Here's the drawing with two shaded views (mm, measured from the low corner). I have some questions. A direction names the side the tool comes from. Coordinates: 2 decimals unless noted, no trailing zeros. Write each loop counter-clockwise with the first axis right and the second up, starting at its lowest first coordinate (ties: lowest second). Pieces come first, ordered by that corner, then holes. Notation, with made-up numbers: M 75.25,-31.75 L 133.25,-31.75 A27 ccw 133.25,4.25 Z; hole C 56,68.5 d3. An arc over 180 degrees is marked long. Answer as CSV lines item,"result". Start each with the question number.
Item 1: Suppose I cut it at A-A, the plane z = 12.5. Write out the boundary of the cut face in (x, y).
Item 2: Suppose I cut it at C-C, the plane y = 9. Write out the boundary of the cut face in (x, z).
Item 3: If I drill on line 1 along X through (y, z) = (35, 15.25); line 2 along Y through (x, z) = (22.5, 8.5), over which ranges is the centre line in solid material (lowest first)? Write a range as [from, to].
Item 4: Suppose I cut it at D-D, the plane x = 22.5. Write out the boundary of the cut face in (y, z).
Item 5: On a 3-axis mill with a long thin cutter (end or side, diameter ignored), from which of +Z, -Z, +X, -X, +Y, -Y can I reach the whole of each face in a straight line? I mean the marked faces 1 and 2. Say none if no direction works.
Item 6: I'm going to push flat-ended pins straight in: P1, Ø17.5, axis at x = 19, y = 19, coming from the +Z side; P2, Ø1, axis at x = 38.5, y = 10, coming from the +Z side. Where does each tip first touch, or does it pass through?
Item 7: Suppose I cut it at B-B, the plane z = 17.5. Write out the boundary of the cut face in (x, y).
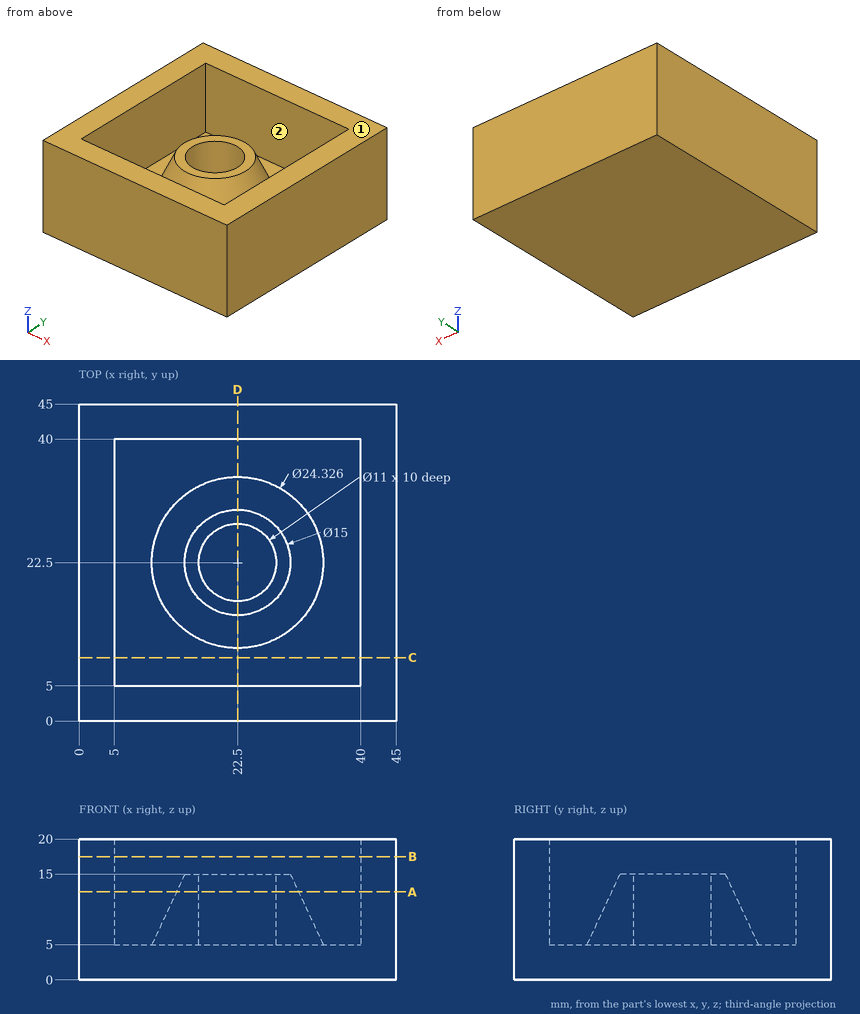
Ans:
1,outline,"M 0,0 L 45,0 L 45,45 L 0,45 Z; C 22.5,22.5 d17.33; hole M 5,5 L 40,5 L 40,40 L 5,40 Z; hole C 22.5,22.5 d11"
2,outline,"M 0,0 L 45,0 L 45,20 L 40,20 L 40,5 L 5,5 L 5,20 L 0,20 Z"
3,line 1,"x = [0, 5], [40, 45]"
3,line 2,"y = [0, 5], [11.97, 17], [28, 33.03], [40, 45]"
4,outline,"M 0,0 L 45,0 L 45,20 L 40,20 L 40,5 L 34.66,5 L 30,15 L 28,15 L 28,5 L 17,5 L 17,15 L 15,15 L 10.34,5 L 5,5 L 5,20 L 0,20 Z"
5,face 1,"+Z, +X, -X, +Y, -Y"
5,face 2,"+Z"
6,P1,"stops at z = 15"
6,P2,"stops at z = 5"
7,outline,"M 0,0 L 45,0 L 45,45 L 0,45 Z; hole M 5,5 L 40,5 L 40,40 L 5,40 Z"
